from build123d import *

# Parameters (mm, degrees)
SKETCH_1_W             = 100
SKETCH_1_H             = 30
EXTRUDE_1_DEPTH        = 50
CUT_EXTRUDE_1_DEPTH    = 50
PATTERN_LINEAR_1_COUNT = 3
PATTERN_LINEAR_1_PITCH = 10


with BuildPart() as part:
    # 草图1 → 凸台-拉伸1 (new body)
    with BuildSketch(Plane(origin=(0, 0, 0), x_dir=(1, 0, 0), z_dir=(0, 1, 0))):
        with Locations((50, 15)):
            Rectangle(SKETCH_1_W, SKETCH_1_H)
    extrude(amount=EXTRUDE_1_DEPTH)

    # 草图2 → 切除-拉伸1 (cut)
    with BuildSketch(Plane(origin=(0, 50, 0), x_dir=(1, 0, 0), z_dir=(0, 1, 0))):
        with BuildLine():
            Line((5, 6.75), (95, 6.75))
            ThreePointArc((95, 6.75), (96.75, 5), (95, 3.25))
            Line((95, 3.25), (5, 3.25))
            ThreePointArc((5, 3.25), (3.25, 5), (5, 6.75))
        make_face()
    cut_extrude_1 = extrude(amount=-CUT_EXTRUDE_1_DEPTH, mode=Mode.SUBTRACT)

    # 阵列(线性)1: 切除-拉伸1 ×3
    with Locations(*[(0, 0, -i * PATTERN_LINEAR_1_PITCH) for i in range(1, PATTERN_LINEAR_1_COUNT)]):
        add(cut_extrude_1, mode=Mode.SUBTRACT)


solid = part.part
Work out the finished part from the listing and answer in its coordinate system (mm). A direction names the side the tool comes from. Round coordinates to 2 decimals unless told otherwise and drop trailing zeros. Loops run counter-clockwise (first coordinate to the right, second up) from the corner with the lowest first, then second, coordinate; pieces in that order, holes last. Notation, with made-up numbers: (-8, 70.25) -> (17, 70.25) arc R16 ccw to (17, 75.25) -> close; hole circle Ø9 at (58, 29). An arc over 180 degrees is marked (long way). Use one line per item in the form item = value.
(1) Find section C-C on y = 23. Give the vertices of the cut face in (x, z), then the cut area to 3 significant figures.
Answer list:
outline = (0, -30) -> (100, -30) -> (100, 0) -> (0, 0) -> close; hole (5, -26.75) -> (95, -26.75) arc R1.75 ccw to (95, -23.25) -> (5, -23.25) arc R1.75 ccw to start; hole (5, -16.75) -> (95, -16.75) arc R1.75 ccw to (95, -13.25) -> (5, -13.25) arc R1.75 ccw to start; hole (5, -6.75) -> (95, -6.75) arc R1.75 ccw to (95, -3.25) -> (5, -3.25) arc R1.75 ccw to start
area = 2,030 mm2
(2) Find section A-A on z = -5. Give the vertices of the cut face in (x, y), then the cut area to 3 significant figures.
Answer list:
outline = (0, 0) -> (3.25, 0) -> (3.25, 50) -> (0, 50) -> close; (96.75, 0) -> (100, 0) -> (100, 50) -> (96.75, 50) -> close
area = 325 mm2
(3) Find section B-B on x = 24. Give the vertices of the cut face in (y, z).
Answer list:
outline = (0, -30) -> (50, -30) -> (50, -26.75) -> (0, -26.75) -> close; (0, -23.25) -> (50, -23.25) -> (50, -16.75) -> (0, -16.75) -> close; (0, -13.25) -> (50, -13.25) -> (50, -6.75) -> (0, -6.75) -> close; (0, -3.25) -> (50, -3.25) -> (50, 0) -> (0, 0) -> close
(4) A flat-ended cylindrical pin translates along its axis: P1, Ø15, axis at x = 43.5, y = 29.5, coming from the +Z side. Find the tip coordinate at first contact, or state that the pin passes through.
Answer list:
P1 = 0
(5) A tool of negligible diameter and unlimited length cuts with its end or side. For faces 4 (the flat face through (51, 25, -23.25)), 5 (the flat face through (0, 25, -15)), from which of +Z, -Z, +X, -X, +Y, -Y can it reach the whole face along a straight path? Write none if from no direction.
Answer list:
face_4 = +Y, -Y
face_5 = +Z, -Z, -X, +Y, -Y
(6) Straight lines are drawn through the part: line 1 (Z direction, x = 56, y = 44); line 2 (X direction, y = 18, z = -4.25); line 3 (X direction, y = 25.5, z = -26.25). For each, find the intervals that lie inside material, in ascending order.
Answer list:
line_1 = -30 to -26.75, -23.25 to -16.75, -13.25 to -6.75, -3.25 to 0
line_2 = 0 to 3.42, 96.58 to 100
line_3 = 0 to 3.78, 96.22 to 100
(7) For a pull along Z with two mould halves and no side action, classify faces 1 (the flat face through (49, 25, -30)), 2 (the flat face through (49, 50, -12)), 3 (the flat face through (49, 25, -6.75)) as released by +Z, released by -Z, zero draft, split by the parting line, or undercut.
Answer list:
face_1 = released by -Z
face_2 = zero draft
face_3 = undercut
